Check sheet for the modelled part. Datum: model origin and axes. Units: mm. Face numbers are marked on the shaded views. A direction names the side the tool comes from. Coordinates: 2 decimals unless noted, no trailing zeros. Order: outer loops, then holes, each group sorted by start corner. A loop starts at its lowest first (then second) coordinate and runs counter-clockwise, first axis right, second up.
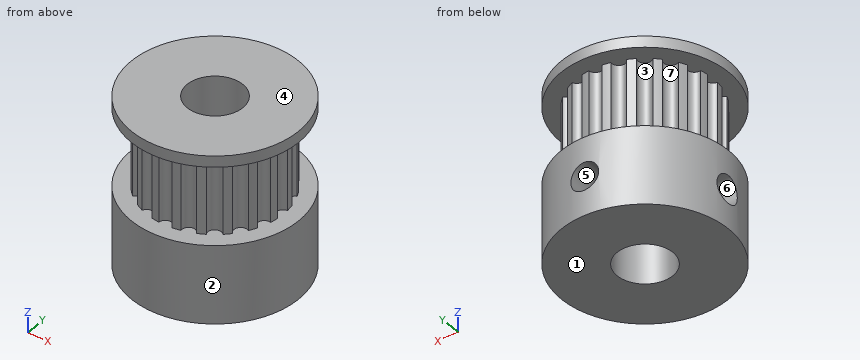
from build123d import *

# Parameters (mm, degrees)
SKETCH_1_R               = 7.5
EXTRUDE_1_DEPTH          = 3.5
SKETCH_2_R               = 6.115
EXTRUDE_2_DEPTH          = 7
CUT_EXTRUDE_3_DEPTH      = 7
SKETCH_3_R               = 7.5
EXTRUDE_3_DEPTH          = 1
SKETCH_6_R               = 2.5
CUT_EXTRUDE_2_DEPTH      = 16
PATTERN_CIRCULAR_2_COUNT = 20
SKETCH_13_W              = 1.25
SKETCH_13_H              = 7.5
PATTERN_CIRCULAR_4_COUNT = 2
PATTERN_CIRCULAR_4_ANGLE = 90


with BuildPart() as part:
    # 草圖1 → 填料-伸長1 (new body, symmetric)
    with BuildSketch(Plane.XY):
        Circle(SKETCH_1_R)
    extrude(amount=EXTRUDE_1_DEPTH, both=True)

    # 草圖2 → 填料-伸長2 (add)
    with BuildSketch(Plane.XY.offset(3.5)):
        Circle(SKETCH_2_R)
    extrude(amount=EXTRUDE_2_DEPTH)

    # 草圖7 → 除料-伸長3 (cut)
    with BuildSketch(Plane.XY.offset(10.5)):
        with BuildLine():
            ThreePointArc((-0.599277509, 6.085564186), (0, 5.515), (0.599277509, 6.085564186))
            ThreePointArc((0.599277509, 6.085564186), (0, 6.115), (-0.599277509, 6.085564186))
        make_face()
    cut_extrude_3 = extrude(amount=-CUT_EXTRUDE_3_DEPTH, mode=Mode.SUBTRACT)

    # 草圖3 → 填料-伸長3 (add)
    with BuildSketch(Plane.XY.offset(10.5)):
        Circle(SKETCH_3_R)
    extrude(amount=EXTRUDE_3_DEPTH)

    # 草圖6 → 除料-伸長2 (cut, through all)
    with BuildSketch(Plane(origin=(0, 0, -3.5), x_dir=(-1, 0, 0), z_dir=(0, 0, -1))):
        Circle(SKETCH_6_R)
    extrude(amount=-CUT_EXTRUDE_2_DEPTH, mode=Mode.SUBTRACT)

    # 環狀複製排列2: 除料-伸長3 ×20 about axis
    pattern_circular_2_axis = Axis((0, 0, 0), (0, 0, 1))
    for i in range(1, PATTERN_CIRCULAR_2_COUNT):
        add(cut_extrude_3.rotate(pattern_circular_2_axis, i * 360 / PATTERN_CIRCULAR_2_COUNT), mode=Mode.SUBTRACT)

    # 草圖13 → M3x0.5 螺紋孔3 (revolve, cut)
    with BuildSketch(Plane(origin=(0, 0, 0), x_dir=(0, 0, -1), z_dir=(1, 0, 0))):
        with Locations((0.625, 3.75)):
            Rectangle(SKETCH_13_W, SKETCH_13_H)
    m3x0_5_3 = revolve(axis=Axis((0, -6.35, 0), (0, 1, 0)), mode=Mode.SUBTRACT)

    # 環狀複製排列4: M3x0.5 螺紋孔3 ×2 about axis
    pattern_circular_4_axis = Axis((0, 0, 3.5), (0, 0, 1))
    for i in range(1, PATTERN_CIRCULAR_4_COUNT):
        add(m3x0_5_3.rotate(pattern_circular_4_axis, i * PATTERN_CIRCULAR_4_ANGLE / (PATTERN_CIRCULAR_4_COUNT - 1)), mode=Mode.SUBTRACT)


solid = part.part
(1) Cross-section at D-D (z = 0). Enter the section's corners in (x, y).
Filled in:
outline: (-7.4, -1.25) arc R7.5 ccw (long way) to (1.25, 7.4) - (1.25, 2.17) arc R2.5 cw (long way) to (-2.17, -1.25) - close; (-7.4, 1.25) - (-2.17, 1.25) arc R2.5 cw to (-1.25, 2.17) - (-1.25, 7.4) arc R7.5 ccw to start
(2) Cross-section at C-C (y = 0). Enter the section's corners in (x, z) (3 decimals), and give its area (3 significant figures).
Filled in:
outline: (-7.5, -3.5) - (-2.5, -3.5) - (-2.5, -1.25) - (-7.5, -1.25) - close; (-7.5, 1.25) - (-2.5, 1.25) - (-2.5, 11.5) - (-7.5, 11.5) - (-7.5, 10.5) - (-5.515, 10.5) - (-5.515, 3.5) - (-7.5, 3.5) - close; (2.5, -3.5) - (7.5, -3.5) - (7.5, 3.5) - (5.515, 3.5) - (5.515, 10.5) - (7.5, 10.5) - (7.5, 11.5) - (2.5, 11.5) - close
area: 110 mm2
(3) Cross-section at A-A (y = 6.75). Enter the section's corners in (x, z).
Filled in:
outline: (-3.27, -3.5) - (3.27, -3.5) - (3.27, 3.5) - (-3.27, 3.5) - close; (-3.27, 10.5) - (3.27, 10.5) - (3.27, 11.5) - (-3.27, 11.5) - close; hole circle Ø2.5 at (0, 0)
(4) Tool access check on the marked faces 4, 5, 6 and 7. Record the directions out of +Z, -Z, +X, -X, +Y, -Y that give a thin tool (end or side, any length) a straight path to the whole face; none if there is none.
Filled in:
face 4: +Z, +X, -X, +Y, -Y
face 5: +Y
face 6: -X
face 7: none
(5) Release check for a two-part mould opening along Y. For the marked faces 1, 2 and 3 record: +Y half, -Y half, draft (parallel to the pull), parting line (faces both ways), or undercut.
Filled in:
face 1: draft
face 2: parting line
face 3: undercut
(6) Go/stop test with flat-tipped pins: P1, Ø1.5, axis at x = 0, z = 0, coming from the +Y side; P2, Ø3, axis at y = 2.5, z = 4.5, coming from the +X side; P3, Ø6, axis at x = -4, z = 4, coming from the -Y side. Record where each tip stops, or that it passes through.
Filled in:
P1: stops at y = -2.38
P2: stops at x = 7.37
P3: stops at y = -7.43
(7) Cross-section at B-B (x = 0). Enter the section's corners in (y, z) (3 decimals).
Filled in:
outline: (-7.5, -3.5) - (-2.5, -3.5) - (-2.5, 11.5) - (-7.5, 11.5) - (-7.5, 10.5) - (-5.515, 10.5) - (-5.515, 3.5) - (-7.5, 3.5) - close; (2.5, -3.5) - (7.5, -3.5) - (7.5, -1.25) - (2.5, -1.25) - close; (2.5, 1.25) - (7.5, 1.25) - (7.5, 3.5) - (5.515, 3.5) - (5.515, 10.5) - (7.5, 10.5) - (7.5, 11.5) - (2.5, 11.5) - close
(8) Thickness scan on probe 1 along Y at (x, z) = (0, 6.25) (3 decimals); probe 2 along Z at (x, y) = (4.5, 4.5); probe 3 along Y at (x, z) = (1.75, 4). Record the ranges inside material, lowest first.
Filled in:
probe 1: y = -5.515 to -2.5, 2.5 to 5.515
probe 2: z = -3.5 to 3.5, 10.5 to 11.5
probe 3: y = -5.23 to -1.79, 1.79 to 5.23
